from build123d import *

# Parameters (mm, degrees)
SKETCH1_W                    = 100
SKETCH1_H                    = 50
BASE_FLANGE1_DEPTH           = 3
SKETCH2_R                    = 11.05
SKETCH2_R_2                  = 1.75
CUT_EXTRUDE1_DEPTH           = 104.121287812
CUT_EXTRUDE3_DEPTH           = 104.121287812
SKETCHED_BEND2_OUTLINE_W     = 3
SKETCHED_BEND2_OUTLINE_H     = 50
SKETCHED_BEND2_DEPTH         = 47.070796327
SKETCHED_START               = 47.411206327
SKETCHED_BEND2_2_OUTLINE_W   = 47.929203673
SKETCHED_BEND2_2_OUTLINE_H   = 50
SKETCHED_BEND2_2_OUTLINE_R   = 1.75
SKETCHED_BEND2_2_OUTLINE_R_2 = 11.05
SKETCHED_BEND2_2_DEPTH       = 2.65959
SKETCHED_START_2             = 47.070796327
SKETCHED_BEND2_3_OUTLINE_W   = 47.929203673
SKETCHED_BEND2_3_OUTLINE_H   = 50
SKETCHED_BEND2_3_OUTLINE_R   = 1.75
SKETCHED_BEND2_3_OUTLINE_R_2 = 11.05
SKETCHED_BEND2_3_DEPTH       = 3.5
SKETCHED_START_3             = -26
SKETCHED_BEND2_4_DEPTH       = 52
BOSS_EXTRUDE1_DEPTH          = 3
CHAMFER1_SIZE                = 5
CHAMFER2_SIZE                = 0.3


with BuildPart() as part:
    # Base-Flange1: sheet metal written as solids
    # Sketch1 → Base-Flange1 (new body)
    with BuildSketch(Plane(origin=(0, 0, 0), x_dir=(1, 0, 0), z_dir=(0, 1, 0))):
        with Locations((50, 0)):
            Rectangle(SKETCH1_W, SKETCH1_H)
    extrude(amount=-BASE_FLANGE1_DEPTH)

    # Sketch2 → Cut-Extrude1 (cut, through all)
    with BuildSketch(Plane(origin=(0, 0, 0), x_dir=(1, 0, 0), z_dir=(0, 1, 0))):
        with Locations(Location((21, 0, 0), (0, 0, 270))):
            Circle(SKETCH2_R)
        with Locations(Location((5.5, 15.5, 0), (0, 0, 270))):
            Circle(SKETCH2_R_2)
        with Locations(Location((36.5, 15.5, 0), (0, 0, 270))):
            Circle(SKETCH2_R_2)
        with Locations(Location((36.5, -15.5, 0), (0, 0, 270))):
            Circle(SKETCH2_R_2)
        with Locations(Location((5.5, -15.5, 0), (0, 0, 270))):
            Circle(SKETCH2_R_2)
    extrude(amount=-CUT_EXTRUDE1_DEPTH, mode=Mode.SUBTRACT)

    # Sketch4 → Cut-Extrude3 (cut, through all)
    with BuildSketch(Plane(origin=(0, 0, 0), x_dir=(1, 0, 0), z_dir=(0, 1, 0))):
        with BuildLine():
            Line((59, 17.1), (89, 17.1))
            ThreePointArc((89, 17.1), (91.1, 15), (89, 12.9))
            Line((89, 12.9), (59, 12.9))
            ThreePointArc((59, 12.9), (56.9, 15), (59, 17.1))
        make_face()
        with BuildLine():
            Line((59, -12.9), (89, -12.9))
            ThreePointArc((89, -12.9), (91.1, -15), (89, -17.1))
            Line((89, -17.1), (59, -17.1))
            ThreePointArc((59, -17.1), (56.9, -15), (59, -12.9))
        make_face()
    extrude(amount=-CUT_EXTRUDE3_DEPTH, mode=Mode.SUBTRACT)

    # Sketched Bend2: read off the stored shape, not the designer's step
    # Sketched Bend2 outline → Sketched Bend2 (cut)
    with BuildSketch(Plane.YZ):
        with Locations((-1.5, 0)):
            Rectangle(SKETCHED_BEND2_OUTLINE_W, SKETCHED_BEND2_OUTLINE_H)
    extrude(amount=SKETCHED_BEND2_DEPTH, mode=Mode.SUBTRACT)

    # Sketched Bend2 2 outline → Sketched Bend2 2 (add)
    with BuildSketch(Plane.YZ.offset(SKETCHED_START)):
        with Locations((23.964601837, 0)):
            Rectangle(SKETCHED_BEND2_2_OUTLINE_W, SKETCHED_BEND2_2_OUTLINE_H)
        with Locations((11.429203673, -15.5)):
            Circle(SKETCHED_BEND2_2_OUTLINE_R, mode=Mode.SUBTRACT)
        with Locations((42.429203673, -15.5)):
            Circle(SKETCHED_BEND2_2_OUTLINE_R, mode=Mode.SUBTRACT)
        with Locations((11.429203673, 15.5)):
            Circle(SKETCHED_BEND2_2_OUTLINE_R, mode=Mode.SUBTRACT)
        with Locations((26.929203673, 0)):
            Circle(SKETCHED_BEND2_2_OUTLINE_R_2, mode=Mode.SUBTRACT)
        with Locations((42.429203673, 15.5)):
            Circle(SKETCHED_BEND2_2_OUTLINE_R, mode=Mode.SUBTRACT)
    extrude(amount=SKETCHED_BEND2_2_DEPTH)

    # Sketched Bend2 3 outline → Sketched Bend2 3 (add)
    with BuildSketch(Plane.YZ.offset(SKETCHED_START_2)):
        with Locations((23.964601837, 0)):
            Rectangle(SKETCHED_BEND2_3_OUTLINE_W, SKETCHED_BEND2_3_OUTLINE_H)
        with Locations((11.429203673, -15.5)):
            Circle(SKETCHED_BEND2_3_OUTLINE_R, mode=Mode.SUBTRACT)
        with Locations((42.429203673, -15.5)):
            Circle(SKETCHED_BEND2_3_OUTLINE_R, mode=Mode.SUBTRACT)
        with Locations((11.429203673, 15.5)):
            Circle(SKETCHED_BEND2_3_OUTLINE_R, mode=Mode.SUBTRACT)
        with Locations((26.929203673, 0)):
            Circle(SKETCHED_BEND2_3_OUTLINE_R_2, mode=Mode.SUBTRACT)
        with Locations((42.429203673, 15.5)):
            Circle(SKETCHED_BEND2_3_OUTLINE_R, mode=Mode.SUBTRACT)
    extrude(amount=SKETCHED_BEND2_3_DEPTH)

    # Sketched Bend2 4 outline → Sketched Bend2 4 (cut)
    with BuildSketch(Plane.XY.offset(SKETCHED_START_3)):
        with BuildLine():
            Line((50.570796327, 47.929203673), (50.070796327, 47.929203673))
            Line((50.070796327, 47.929203673), (50.070796327, 0.5))
            ThreePointArc((50.070796327, 0.5), (50.217242936, 0.146446609), (50.570796327, 0))
            Line((50.570796327, 0), (50.570796327, 47.929203673))
        make_face()
        with BuildLine():
            ThreePointArc((50.570796327, -3), (48.095922593, -1.974873734), (47.070796327, 0.5))
            Line((47.070796327, 0.5), (47.070796327, -3))
            Line((47.070796327, -3), (50.570796327, -3))
        make_face()
    extrude(amount=SKETCHED_BEND2_4_DEPTH, mode=Mode.SUBTRACT)

    # Sketch6 → Boss-Extrude1 (add)
    with BuildSketch(Plane.XY.offset(25)):
        Polygon((50.070796327, 30), (75.070796327, 0), (50.070796327, 0), align=None)
    boss_extrude1 = extrude(amount=-BOSS_EXTRUDE1_DEPTH)

    # Mirror1: Boss-Extrude1 across plane
    add(boss_extrude1.mirror(Plane.XY))

    # Chamfer1
    chamfer1_edges = [part.edges().sort_by_distance(p)[0] for p in [
        (48.570796327, 47.929203673, -25),
        (48.570796327, 47.929203673, 25),
        (100, -1.5, -25),
        (100, -1.5, 25),
    ]]
    chamfer(chamfer1_edges, length=CHAMFER1_SIZE)

    # Chamfer2
    chamfer2_edges = [part.edges().sort_by_distance(p)[0] for p in [
        (47.070796327, 15.879203673, 0),
        (50.070796327, 15.879203673, 0),
        (47.070796327, 40.679203673, -15.5),
        (50.070796327, 40.679203673, -15.5),
        (47.070796327, 9.679203673, -15.5),
        (50.070796327, 9.679203673, -15.5),
        (47.070796327, 9.679203673, 15.5),
        (50.070796327, 9.679203673, 15.5),
        (47.070796327, 40.679203673, 15.5),
        (50.070796327, 40.679203673, 15.5),
        (74, 0, -17.1),
        (91.1, 0, -15),
        (74, 0, -12.9),
        (56.9, 0, -15),
        (74, 0, 12.9),
        (91.1, 0, 15),
        (74, 0, 17.1),
        (56.9, 0, 15),
        (56.9, -3, 15),
        (74, -3, 17.1),
        (91.1, -3, 15),
        (74, -3, 12.9),
        (56.9, -3, -15),
        (74, -3, -12.9),
        (91.1, -3, -15),
        (74, -3, -17.1),
    ]]
    chamfer(chamfer2_edges, length=CHAMFER2_SIZE)


solid = part.part
Here's how the part is built. I have some questions about the finished solid (model axes, mm). A direction names the side the tool comes from. Round coordinates to 2 decimals unless told otherwise and drop trailing zeros. Write each loop counter-clockwise with the first axis right and the second up, starting at its lowest first coordinate (ties: lowest second). Pieces come first, ordered by that corner, then holes.
1. Suppose I cut it at C-C (y = 1.5). List the corners of the cut face in (x, z) for me.
2. If we mould it in two halves opening along Y, with no side actions, what happens to faces 1 (the cylindrical face through (48.554, 11.201, -13.765)), 2 (the conical face through (91.21, -0.19, 14.95)), 3 (the cylindrical face through (91.1, -1.5, -15))? For each: released by +Y, released by -Y, zero draft, split by the parting line, or undercut.
3. Will these pins go through, and if not, where does the flat tip stop? pin 1 Ø13.5 at (y, z) = (26.93, 0) entering from +X; pin 2 Ø2 at (x, z) = (93, 18.5) entering from +Y; pin 3 Ø2 at (y, z) = (27.5, -20) entering from +X; pin 4 Ø8 at (y, z) = (14, 19) entering from +X.
4. Suppose I cut it at D-D (z = 15.5). State how many separate pieces and enclosed holes the cut face has, and give its area (3 significant figures).
5. Suppose I cut it at A-A (z = 0). List the corners of the cut face in (x, y) for me.
6. I need wall thicknesses on L1, parallel to Y at x = 48.25, z = 15.5; L2, parallel to Y at x = 48.05, z = -15.5; L3, parallel to Z at x = 56, y = 19. Which ranges of each line are inside material? Lowest first, please.
7. For faces 4 (the flat face through (74, -1, 12.9)), 5 (the flat face through (75, 0, 0)), 6 (the conical face through (56.79, -2.81, -15.05)), which set-ups out of +Z, -Z, +X, -X, +Y, -Y let a thin tool reach every point of the face, with its end or its side?
8. Suppose I cut it at B-B (x = 78). List the corners of the cut face in (y, z) for me, and give its area (3 significant figures).
Answer sheet:
1. outline: (47.07, -25) - (73.82, -25) - (73.82, -22) - (50.07, -22) - (50.07, 22) - (73.82, 22) - (73.82, 25) - (47.07, 25) - close
2. face 1: undercut
2. face 2: released by +Y
2. face 3: zero draft
3. pin 1: passes through
3. pin 2: stops at y = 0
3. pin 3: stops at x = 50.07
3. pin 4: stops at x = 65.61
4. separate pieces: 4
4. enclosed holes: 0
4. area: 176 mm2
5. outline: (47.07, 0.5) arc R3.5 ccw to (50.57, -3) - (100, -3) - (100, 0) - (50.57, 0) arc R0.5 cw to (50.07, 0.5) - (50.07, 15.58) - (49.77, 15.88) - (47.37, 15.88) - (47.07, 15.58) - close; (47.07, 38.28) - (47.37, 37.98) - (49.77, 37.98) - (50.07, 38.28) - (50.07, 47.93) - (47.07, 47.93) - close
6. L1: y = -2.12 to 9.68, 13.18 to 40.68, 44.18 to 47.93
6. L2: y = -1.93 to 9.68, 13.18 to 40.68, 44.18 to 47.93
6. L3: z = -25 to -22, 22 to 25
7. face 4: +Y, -Y
7. face 5: +X, +Y
7. face 6: -Y
8. outline: (-3, -25) - (0, -25) - (0, -17.4) - (-0.3, -17.1) - (-2.7, -17.1) - (-3, -17.4) - close; (-3, -12.6) - (-2.7, -12.9) - (-0.3, -12.9) - (0, -12.6) - (0, 12.6) - (-0.3, 12.9) - (-2.7, 12.9) - (-3, 12.6) - close; (-3, 17.4) - (-2.7, 17.1) - (-0.3, 17.1) - (0, 17.4) - (0, 25) - (-3, 25) - close
8. area: 124 mm2
